For this review, take the finished solid that the model builds, in its own axes (mm). Face numbers are marked on the shaded views. A direction names the side the tool comes from. Round coordinates to 2 decimals unless told otherwise and drop trailing zeros. Order: outer loops, then holes, each group sorted by start corner. A loop starts at its lowest first (then second) coordinate and runs counter-clockwise, first axis right, second up. Notation, with made-up numbers: M -23.5,88.5 L -4.5,88.5 A24 cw -4.5,119.5 Z; hole C 9,82 d3. An arc over 180 degrees is marked long. Answer as a JSON object with one key per item and string values.
from build123d import *

# Parameters (mm, degrees)
SKETCH_1_R      = 12
SKETCH_1_R_2    = 2.1
EXTRUDE_1_DEPTH = 3
EXTRUDE_START   = -2
EXTRUDE_2_DEPTH = 2


with BuildPart() as part:
    # 草图1 → 凸台-拉伸1 (new body)
    with BuildSketch(Plane.XY):
        Circle(SKETCH_1_R)
        with Locations((0, 6)):
            Circle(SKETCH_1_R_2, mode=Mode.SUBTRACT)
        with Locations((6, 0)):
            Circle(SKETCH_1_R_2, mode=Mode.SUBTRACT)
        with Locations((0, -6)):
            Circle(SKETCH_1_R_2, mode=Mode.SUBTRACT)
        with Locations((-6, 0)):
            Circle(SKETCH_1_R_2, mode=Mode.SUBTRACT)
    extrude(amount=EXTRUDE_1_DEPTH)

    # 草图2 → 凸台-拉伸2 (add)
    with BuildSketch(Plane.XY.offset(3).offset(EXTRUDE_START)):
        with BuildLine():
            Line((-11.326666422, 13.989518497), (-10.233844137, 6.266453079))
            ThreePointArc((-10.233844137, 6.266453079), (-7.551110948, 9.326345664), (-4, 11.313708499))
            Line((-4, 11.313708499), (-11.326666422, 13.989518497))
        make_face()
        with BuildLine():
            Line((11.326666422, 13.989518497), (4, 11.313708499))
            ThreePointArc((4, 11.313708499), (7.551110948, 9.326345664), (10.233844137, 6.266453079))
            Line((10.233844137, 6.266453079), (11.326666422, 13.989518497))
        make_face()
    extrude(amount=EXTRUDE_2_DEPTH)


solid = part.part
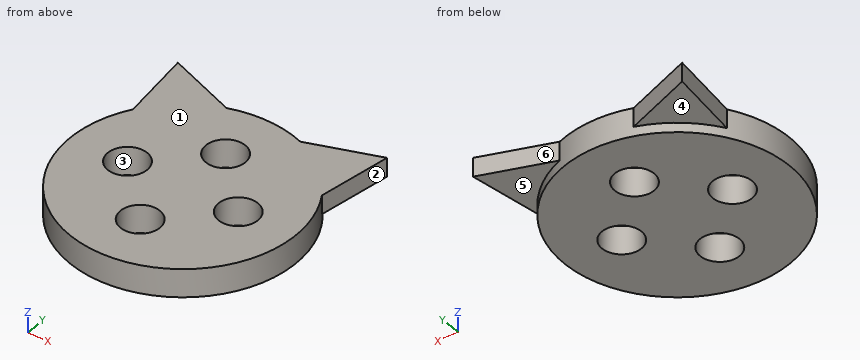
1) For L1, parallel to Y at x = 0, z = 2.8; L2, parallel to X at y = -1, z = 1.5; L3, parallel to Y at x = 0.5, z = 2.35, list the stretches that pass through material, from the lowest coordinate up.
Geometry check:
{"L1": "y = -12 to -8.1, -3.9 to 3.9, 8.1 to 12", "L2": "x = -11.96 to -7.85, -4.15 to 4.15, 7.85 to 11.96", "L3": "y = -11.99 to -8.04, -3.96 to 3.96, 8.04 to 11.99"}
2) Machinability: for the marked faces 4, 5 and 6, which of the approach directions +Z, -Z, +X, -X, +Y, -Y give a long, thin tool a straight path to every point of the face, cutting with its end or side? Answer none if there is none.
Geometry check:
{"face 4": "-Z, -X, +Y", "face 5": "-Z, +X, +Y", "face 6": "+Z, -Z, +Y"}
3) Add section D-D on y = -0.5. State the section outline as (x, z) points.
Geometry check:
{"outline": "M -11.99,0 L -8.04,0 L -8.04,3 L -11.99,3 Z; M -3.96,0 L 3.96,0 L 3.96,3 L -3.96,3 Z; M 8.04,0 L 11.99,0 L 11.99,3 L 8.04,3 Z"}
4) Mouldability with a two-part tool opening along X and no side actions: class the marked faces 1, 2 and 3 as +X half, -X half, draft (parallel to the pull), parting line (faces both ways), or undercut.
Geometry check:
{"face 1": "draft", "face 2": "+X half", "face 3": "undercut"}
5) Add section B-B on z = 2.65. State the section outline as (x, y) points, and give its area (3 significant figures).
Geometry check:
{"outline": "M -11.33,13.99 L -10.23,6.27 A12 ccw long 10.23,6.27 L 11.33,13.99 L 4,11.31 A12 ccw -4,11.31 Z; hole C -6,0 d4.2; hole C 0,-6 d4.2; hole C 0,6 d4.2; hole C 6,0 d4.2", "area": "443 mm²"}
6) Insertion check: P1, Ø3.5, axis at x = -6, y = 10, coming from the -Z side; P2, Ø1, axis at y = 9.5, z = 1, coming from the +X side; P3, Ø3.5, axis at x = 9.5, y = 10, coming from the -Z side. Each pin has a flat end and moves straight along its axis. Give the tip position at first contact, or say it passes through.
Geometry check:
{"P1": "stops at z = 0", "P2": "stops at x = 10.76", "P3": "stops at z = 1"}
7) Add section C-C on y = -6. State the section outline as (x, z) points.
Geometry check:
{"outline": "M -10.39,0 L -2.1,0 L -2.1,3 L -10.39,3 Z; M 2.1,0 L 10.39,0 L 10.39,3 L 2.1,3 Z"}
8) Add section A-A on x = 0. State the section outline as (y, z) points.
Geometry check:
{"outline": "M -12,0 L -8.1,0 L -8.1,3 L -12,3 Z; M -3.9,0 L 3.9,0 L 3.9,3 L -3.9,3 Z; M 8.1,0 L 12,0 L 12,3 L 8.1,3 Z"}
